from build123d import *

# Parameters (mm, degrees)
SKETCH1_R                   = 2.75
BOSS_EXTRUDE1_DEPTH         = 8
POT_START                   = 8
POT_INSERT_DEPTH            = 2.5
MIDDLE_START                = 3
SKETCH7_R                   = 13
SKETCH7_R_2                 = 11
MIDDLE_FLEX_EXT_CANAL_DEPTH = 5
DISTAL_START                = 5.5
DISTAL_FLEX_EXT_CANAL_DEPTH = 2.5
SKETCH3_R                   = 0.8
SCREW_HOLES_DEPTH           = 44.132654063


# Read off the part's stored shape, not the designer's step: Distal Flex_Ext Canal
with BuildPart() as part:
    # Sketch1 → Boss-Extrude1 (new body)
    with BuildSketch(Plane.XY):
        with BuildLine():
            Line((11.5, 10.28125), (11.5, 0))
            ThreePointArc((11.5, 0), (9.471532219, -6.522275479), (4.101725666, -10.743642146))
            Line((4.101725666, -10.743642146), (32, -9))
            ThreePointArc((32, -9), (40.314915793, 3.444150891), (25.636038969, 6.363961031))
            Line((25.636038969, 6.363961031), (22.4, 9.6))
            Line((22.4, 9.6), (11.5, 10.28125))
        make_face()
        with Locations((32, 0)):
            Circle(SKETCH1_R, mode=Mode.SUBTRACT)
    extrude(amount=BOSS_EXTRUDE1_DEPTH)

    # Sketch2 → Pot Insert (cut)
    with BuildSketch(Plane(origin=(28.28760271, 0, 0), x_dir=(1, 0, 0), z_dir=(0, 0, 1)).offset(POT_START)):
        Polygon((10.71239729, 0), (10.71239729, 1.5), (9.21239729, 1.5), (7.71239729, 4.5), (7.71239729, 5.5), (3.71239729, 5.5), (-0.53760271, 5.5), (-0.53760271, 4.5), (-5.78760271, 4.5), (-5.78760271, 0), (-5.78760271, -4.5), (-0.53760271, -4.5), (-0.53760271, -5.5), (3.71239729, -5.5), (7.71239729, -5.5), (7.71239729, -4.5), (9.21239729, -1.5), (10.71239729, -1.5), align=None)
    extrude(amount=-POT_INSERT_DEPTH, mode=Mode.SUBTRACT)

    # Sketch7 → Middle Flex_Ext Canal (cut)
    # profile 1 of 10: a face of its own
    with BuildSketch(Plane.XY.offset(MIDDLE_START)):
        Circle(SKETCH7_R)
        Circle(SKETCH7_R_2, mode=Mode.SUBTRACT)
    # profile 2 of 10: a face of its own
    with BuildSketch(Plane.XY.offset(MIDDLE_START)):
        with BuildLine():
            Line((19, -2.5), (19, 2.5))
            ThreePointArc((19, 2.5), (17, 0.5), (15, 2.5))
            Line((15, 2.5), (15, 1.5))
            Line((15, 1.5), (12.91317157, 1.5))
            ThreePointArc((12.91317157, 1.5), (12.978274739, 0.751255479), (13, 0))
            ThreePointArc((13, 0), (12.978274739, -0.751255479), (12.91317157, -1.5))
            Line((12.91317157, -1.5), (15, -1.5))
            Line((15, -1.5), (15, -2.5))
            ThreePointArc((15, -2.5), (17, -0.5), (19, -2.5))
        make_face()
    # profile 3 of 10: a face of its own
    with BuildSketch(Plane.XY.offset(MIDDLE_START)):
        with BuildLine():
            ThreePointArc((15, 2.5), (17, 0.5), (19, 2.5))
            ThreePointArc((19, 2.5), (17, 4.5), (15, 2.5))
        make_face()
    # profile 4 of 10: a face of its own
    with BuildSketch(Plane.XY.offset(MIDDLE_START)):
        with BuildLine():
            ThreePointArc((15, -2.5), (17, -4.5), (19, -2.5))
            ThreePointArc((19, -2.5), (17, -0.5), (15, -2.5))
        make_face()
    # profile 5 of 10: a face of its own
    with BuildSketch(Plane.XY.offset(MIDDLE_START)):
        with BuildLine():
            ThreePointArc((15, -2.5), (17, -4.5), (19, -2.5))
            ThreePointArc((19, -2.5), (17, -0.5), (15, -2.5))
        make_face()
    # profile 6 of 10: a face of its own
    with BuildSketch(Plane.XY.offset(MIDDLE_START)):
        with BuildLine():
            ThreePointArc((15, -2.5), (17, -4.5), (19, -2.5))
            ThreePointArc((19, -2.5), (17, -0.5), (15, -2.5))
        make_face()
    # profile 7 of 10: a face of its own
    with BuildSketch(Plane.XY.offset(MIDDLE_START)):
        with BuildLine():
            ThreePointArc((15, -2.5), (17, -4.5), (19, -2.5))
            ThreePointArc((19, -2.5), (17, -0.5), (15, -2.5))
        make_face()
    # profile 8 of 10: a face of its own
    with BuildSketch(Plane.XY.offset(MIDDLE_START)):
        with BuildLine():
            ThreePointArc((15, 2.5), (17, 0.5), (19, 2.5))
            ThreePointArc((19, 2.5), (17, 4.5), (15, 2.5))
        make_face()
    # profile 9 of 10: a face of its own
    with BuildSketch(Plane.XY.offset(MIDDLE_START)):
        with BuildLine():
            ThreePointArc((15, 2.5), (17, 0.5), (19, 2.5))
            ThreePointArc((19, 2.5), (17, 4.5), (15, 2.5))
        make_face()
    # profile 10 of 10: a face of its own
    with BuildSketch(Plane.XY.offset(MIDDLE_START)):
        with BuildLine():
            ThreePointArc((15, 2.5), (17, 0.5), (19, 2.5))
            ThreePointArc((19, 2.5), (17, 4.5), (15, 2.5))
        make_face()
    extrude(amount=MIDDLE_FLEX_EXT_CANAL_DEPTH, mode=Mode.SUBTRACT)

    # Distal Flex_Ext Canal outline → Distal Flex_Ext Canal (cut)
    with BuildSketch(Plane.XY.offset(DISTAL_START)):
        with BuildLine():
            Line((26.223253078, -9.361046683), (32, -9))
            ThreePointArc((32, -9), (28.555849109, -8.314915793), (25.636038969, -6.363961031))
            Line((25.636038969, -6.363961031), (25.193650814, -5.921572875))
            ThreePointArc((25.193650814, -5.921572875), (23.895957419, -5.05448187), (22.365223689, -4.75))
            Line((22.365223689, -4.75), (14.120057685, -4.75))
            ThreePointArc((14.120057685, -4.75), (13.041658829, -4.823017226), (11.982945395, -5.040736023))
            ThreePointArc((11.982945395, -5.040736023), (10.789241938, -7.252052013), (9.192388156, -9.192388156))
            Line((9.192388156, -9.192388156), (9.877416998, -8.507359313))
            ThreePointArc((9.877416998, -8.507359313), (11.823957091, -7.206722805), (14.120057685, -6.75))
            Line((14.120057685, -6.75), (22.365223689, -6.75))
            ThreePointArc((22.365223689, -6.75), (23.130590554, -6.902240935), (23.779437252, -7.335786438))
            Line((23.779437252, -7.335786438), (24.221825407, -7.778174593))
            ThreePointArc((24.221825407, -7.778174593), (25.176485852, -8.627841831), (26.223253078, -9.361046683))
        make_face()
        with BuildLine():
            Line((25.193650814, 5.921572875), (25.636038969, 6.363961031))
            Line((25.636038969, 6.363961031), (24.221825407, 7.778174593))
            Line((24.221825407, 7.778174593), (23.779437252, 7.335786438))
            ThreePointArc((23.779437252, 7.335786438), (23.130590554, 6.902240935), (22.365223689, 6.75))
            Line((22.365223689, 6.75), (14.120057685, 6.75))
            ThreePointArc((14.120057685, 6.75), (12.77586157, 6.902510213), (11.5, 7.352287732))
            Line((11.5, 7.352287732), (11.5, 6.062177826))
            ThreePointArc((11.5, 6.062177826), (11.752574907, 5.556706133), (11.982945395, 5.040736023))
            ThreePointArc((11.982945395, 5.040736023), (13.041658829, 4.823017226), (14.120057685, 4.75))
            Line((14.120057685, 4.75), (22.365223689, 4.75))
            ThreePointArc((22.365223689, 4.75), (23.895957419, 5.05448187), (25.193650814, 5.921572875))
        make_face()
    extrude(amount=DISTAL_FLEX_EXT_CANAL_DEPTH, mode=Mode.SUBTRACT)

    # Sketch3 → Screw Holes (cut, through all)
    with BuildSketch(Plane.XY):
        with Locations((17, 8)):
            Circle(SKETCH3_R)
        with Locations((17, -8)):
            Circle(SKETCH3_R)
        with Locations((17, 2.5)):
            Circle(SKETCH3_R)
        with Locations((17, -2.5)):
            Circle(SKETCH3_R)
    extrude(amount=SCREW_HOLES_DEPTH, mode=Mode.SUBTRACT)


solid = part.part
Geometry check sheet. Reference: the model listing, model coordinates, mm. A direction names the side the tool comes from. Give positions to 0.01 mm unless a question says otherwise; leave off trailing zeros. Order: outer loops, then holes, each group sorted by start corner. A loop starts at its lowest first (then second) coordinate and runs counter-clockwise, first axis right, second up. Notation, with made-up numbers: M -7,-26.5 L 12,-26.5 A21 cw 12,6.5 Z; hole C 4.5,-12.75 d1. An arc over 180 degrees is marked long. Use a Markdown table: item, result.
Item 1: Section check D-D (x = 38.5). Record the cut outline in (y, z).
Answers follow:
| item | result |
|---|---|
| outline | M -6.22,0 L 6.22,0 L 6.22,8 L 1.5,8 L 1.5,5.5 L -1.5,5.5 L -1.5,8 L -6.22,8 Z |
Item 2: Section check B-B (z = 4). Record the cut outline in (x, y).
Answers follow:
| item | result |
|---|---|
| outline | M 7.63,-10.52 L 32,-9 A9 ccw long 25.64,6.36 L 22.4,9.6 L 11.5,10.28 L 11.5,6.06 A13 cw 12.91,1.5 L 15,1.5 L 15,2.5 A2 cw 19,2.5 L 19,-2.5 A2 cw 15,-2.5 L 15,-1.5 L 12.91,-1.5 A13 cw Z; hole C 17,-8 d1.6; hole C 17,8 d1.6; hole C 32,0 d5.5 |
Item 3: Depth check by flat-ended pin: P1, Ø1, axis at x = 17, y = -2.5, coming from the -Z side; P2, Ø10, axis at x = 30, y = -5, coming from the -Z side; P3, Ø2, axis at x = 30.5, z = 6.5, coming from the +Y side; P4, Ø1.4, axis at x = 18, y = -6, coming from the +Z side. Enter the tip coordinate at first touch or a pass-through.
Answers follow:
| item | result |
|---|---|
| P1 | passes through |
| P2 | stops at z = 0 |
| P3 | stops at y = 8.99 |
| P4 | stops at z = 5.5 |
Item 4: Tool access check on faces 1 (the cylindrical face through (23.916, -5.063, 6.732)), 2 (the cylindrical face through (16.41, 8.54, 3.94)), 3 (the flat face through (18, 6.75, 7)). Record the directions out of +Z, -Z, +X, -X, +Y, -Y that give a thin tool (end or side, any length) a straight path to the whole face; none if there is none.
Answers follow:
| item | result |
|---|---|
| face 1 | +Z |
| face 2 | +Z, -Z |
| face 3 | +Z, -X |
Item 5: Section check C-C (x = 17). State how many separate pieces and enclosed holes the cut face has, and give its area (3 significant figures).
Answers follow:
| item | result |
|---|---|
| separate pieces | 5 |
| enclosed holes | 0 |
| area | 68.8 mm2 |
Item 6: Section check A-A (z = 1.5). Record the cut outline in (x, y).
Answers follow:
| item | result |
|---|---|
| outline | M 4.1,-10.74 L 32,-9 A9 ccw long 25.64,6.36 L 22.4,9.6 L 11.5,10.28 L 11.5,0 A11.5 cw Z; hole C 17,-8 d1.6; hole C 17,-2.5 d1.6; hole C 17,2.5 d1.6; hole C 17,8 d1.6; hole C 32,0 d5.5 |
Item 7: Material ranges on line 1 along Y through (x, z) = (17, 0.8); line 2 along Y through (x, z) = (21, 7); line 3 along Y through (x, z) = (17, 3.5), recorded low to high.
Answers follow:
| item | result |
|---|---|
| line 1 | y = -9.94 to -8.8, -7.2 to -3.3, -1.7 to 1.7, 3.3 to 7.2, 8.8 to 9.94 |
| line 2 | y = -9.69 to -6.75, -4.75 to 4.75, 6.75 to 9.69 |
| line 3 | y = -9.94 to -8.8, -7.2 to -4.5, 4.5 to 7.2, 8.8 to 9.94 |
